```python
from build123d import *

# Parameters (mm, degrees)
F0_W      = 400
F0_H      = 280
F1_DEPTH  = 25
F2_W      = 366
F2_H      = 246
F3_DEPTH  = 4
F4_W      = 30
F4_H      = 5
F4_W_2    = 20
F5_DEPTH  = 2
F7_DEPTH  = 300
F8_W      = 75
F8_H      = 238.0099048197
F8_W_2    = 175
F9_DEPTH  = 15
F11_DEPTH = 300
F13_DEPTH = 300


with BuildPart() as f1:
    # F0 (on Top) → F1 (new body)
    with BuildSketch(Plane.XY):
        with Locations((-200, 140)):
            Rectangle(F0_W, F0_H)
    extrude(amount=F1_DEPTH)

    # F2 (on face) → F3 (cut)
    with BuildSketch(Plane.XY.offset(25)):
        with Locations((-200, 140)):
            Rectangle(F2_W, F2_H)
    extrude(amount=-F3_DEPTH, mode=Mode.SUBTRACT)

    # F4 (on face) → F5 (join)
    with BuildSketch(Plane.XY.offset(25)):
        with Locations((-37, 5.5)):
            Rectangle(F4_W, F4_H)
        with Locations((-177, 5.5)):
            Rectangle(F4_W_2, F4_H)
        with Locations((-150, 5.5)):
            Rectangle(F4_W_2, F4_H)
        with Locations((-123, 5.5)):
            Rectangle(F4_W_2, F4_H)
        with Locations((-96, 5.5)):
            Rectangle(F4_W_2, F4_H)
        with Locations((-69, 5.5)):
            Rectangle(F4_W_2, F4_H)
    extrude(amount=F5_DEPTH)

    # F6 (on face) → F7 (join)
    with BuildSketch(Plane.YZ):
        Polygon((140, 0), (125, 0), (-93.7821996545, -58.6225137157), (-89.8999139779, -73.1114011101), (140, -11.5099048197), align=None)
    extrude(amount=-F7_DEPTH)

    # F8 (on face) → F9 (cut)
    with BuildSketch(Plane(origin=(0, 12.25569794, -45.7388873943), x_dir=(1, 0, 0), z_dir=(0, 0.2588190451, -0.9659258263))):
        with Locations((-262.5, -13.245680696)):
            Rectangle(F8_W, F8_H)
        with Locations((-87.5, -13.245680696)):
            Rectangle(F8_W_2, F8_H)
    extrude(amount=-F9_DEPTH, mode=Mode.SUBTRACT)

    # F10 (on face) → F11 (cut)
    with BuildSketch(Plane.YZ):
        Polygon((136.9159302986, 0), (140, -11.5099048197), (140, 0), align=None)
    extrude(amount=-F11_DEPTH, mode=Mode.SUBTRACT)

    # F12 (on face) → F13 (join)
    with BuildSketch(Plane.YZ):
        Polygon((136.1177143235, 2.9789825747), (125, 0), (136.9159302986, 0), align=None)
    extrude(amount=-F13_DEPTH)


solid = f1.part
```
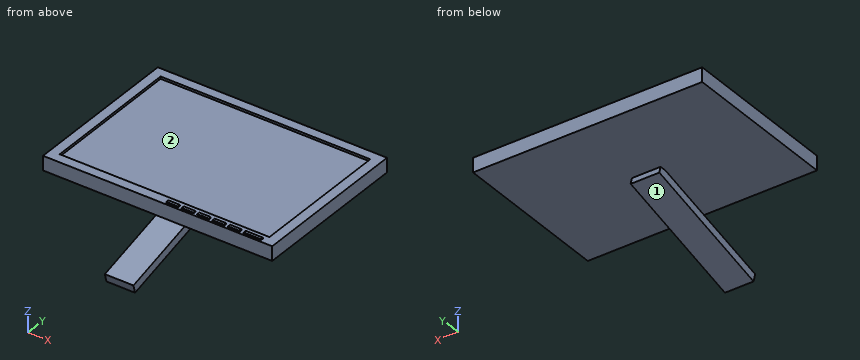
Here's how the part is built. I have some questions about the finished solid (model axes, mm). Face numbers are marked on the shaded views. Give positions to 0.01 mm unless a question says otherwise; leave off trailing zeros. Write each loop counter-clockwise with the first axis right and the second up, starting at its lowest first coordinate (ties: lowest second). Pieces come first, ordered by that corner, then holes. Notation, with made-up numbers: (71, 10.25) -> (123, 10.25) arc R35 cw to (123, 49.25) -> close; hole circle Ø8 at (76.25, -27.5). An arc over 180 degrees is marked (long way). Write each question's results on one line, items separated by ' | '.
Item 1: Suppose I cut it at B-B on y = 166. Write out the boundary of the cut face in (x, z), plus the area to 3 significant figures.
Output:
outline: (-400, 0) -> (0, 0) -> (0, 25) -> (-17, 25) -> (-17, 21) -> (-383, 21) -> (-383, 25) -> (-400, 25) -> close | area: 8,540 mm^2
Item 2: For pin 1 Ø1 at (x, z) = (-120.5, 26) entering from -Y; pin 2 Ø0.6 at (x, z) = (-68.5, 26) entering from +Y; pin 3 Ø3 at (x, z) = (-340.5, -1) entering from -Y; pin 4 Ø1.6 at (x, z) = (-173.5, 25.5) entering from +Y, each with a flat end and sliding along its axis, tell me the tip position at first contact or that it passes through.
Output:
pin 1: stops at y = 3 | pin 2: stops at y = 8 | pin 3: stops at y = 0 | pin 4: stops at y = 280
Item 3: Suppose I cut it at C-C on z = 12.5. Write out the boundary of the cut face in (x, y).
Output:
outline: (-400, 0) -> (0, 0) -> (0, 280) -> (-400, 280) -> close
Item 4: Suppose I cut it at A-A on x = -266. Write out the boundary of the cut face in (y, z).
Output:
outline: (0, 0) -> (280, 0) -> (280, 25) -> (263, 25) -> (263, 21) -> (17, 21) -> (17, 25) -> (0, 25) -> close
Item 5: If I drill on L1, parallel to Z at x = -273.5, y = 97.5; L2, parallel to Y at x = -106, z = 10.5; L3, parallel to X at y = 26, z = -32.5, over which ranges is the centre line in solid material (lowest first)?
Output:
L1: z = 0 to 21 | L2: y = 0 to 280 | L3: x = -225 to -175
Item 6: Suppose I cut it at D-D on x = -28.5. Write out the boundary of the cut face in (y, z).
Output:
outline: (0, 0) -> (280, 0) -> (280, 25) -> (263, 25) -> (263, 21) -> (17, 21) -> (17, 25) -> (8, 25) -> (8, 27) -> (3, 27) -> (3, 25) -> (0, 25) -> close
Item 7: We'd pull the mould along X, two halves only. Please class the marked faces 1 and 2: pulls with the +X half, pulls with the -X half, needs draft (parallel to the pull), parting line crosses it, or undercut.
Output:
face 1: needs draft | face 2: undercut
